Build history of the part. All positions in model axes, mm. A direction names the side the tool comes from. Round coordinates to 2 decimals unless told otherwise and drop trailing zeros. Order: outer loops, then holes, each group sorted by start corner. A loop starts at its lowest first (then second) coordinate and runs counter-clockwise, first axis right, second up. Notation, with made-up numbers: (-34.5, 43.25) -> (-11.5, 43.25) arc R30 cw to (-11.5, 75.25) -> close; hole circle Ø7 at (-23.75, 33). An arc over 180 degrees is marked (long way). Answer as a JSON object with one key per item and string values.
from build123d import *

# Parameters (mm, degrees)
F0_R     = 2.9
F1_DEPTH = 10
F2_W     = 29.9
F2_H     = 90
F3_DEPTH = 40
F4_W     = 7.6
F4_H     = 90
F5_DEPTH = 25
F6_R     = 3.4
F7_DEPTH = 30
F8_SIZE2 = 4
F8_SIZE  = 3


with BuildPart() as f1:
    # F0 (on Right) → F1 (new body)
    with BuildSketch(Plane.YZ):
        with BuildLine():
            Line((-75, -45), (75, -45))
            ThreePointArc((75, -45), (78.535534, -43.535534), (80, -40))
            Line((80, -40), (80, -10))
            ThreePointArc((80, -10), (78.535534, -6.464466), (75, -5))
            Line((75, -5), (45, -5))
            ThreePointArc((45, -5), (41.464466, -3.535534), (40, 0))
            Line((40, 0), (40, 40))
            ThreePointArc((40, 40), (38.535534, 43.535534), (35, 45))
            Line((35, 45), (-35, 45))
            ThreePointArc((-35, 45), (-38.535534, 43.535534), (-40, 40))
            Line((-40, 40), (-40, 0))
            ThreePointArc((-40, 0), (-41.464466, -3.535534), (-45, -5))
            Line((-45, -5), (-75, -5))
            ThreePointArc((-75, -5), (-78.535534, -6.464466), (-80, -10))
            Line((-80, -10), (-80, -40))
            ThreePointArc((-80, -40), (-78.535534, -43.535534), (-75, -45))
        make_face()
        with Locations((-65, -25)):
            Circle(F0_R, mode=Mode.SUBTRACT)
        with Locations((-25, -25)):
            Circle(F0_R, mode=Mode.SUBTRACT)
        with Locations((25, -25)):
            Circle(F0_R, mode=Mode.SUBTRACT)
        with Locations((65, -25)):
            Circle(F0_R, mode=Mode.SUBTRACT)
        with Locations((-25, 25)):
            Circle(F0_R, mode=Mode.SUBTRACT)
        with Locations((25, 25)):
            Circle(F0_R, mode=Mode.SUBTRACT)
    extrude(amount=F1_DEPTH)

    # F2 (on face) → F3 (join)
    with BuildSketch(Plane(origin=(0, 0, 0), x_dir=(0, -1, 0), z_dir=(-1, 0, 0))):
        Rectangle(F2_W, F2_H)
    extrude(amount=F3_DEPTH)

    # F4 (on face) → F5 (cut)
    with BuildSketch(Plane(origin=(-40, 0, 0), x_dir=(0, -1, 0), z_dir=(-1, 0, 0))):
        with Locations((-11.15, 0)):
            Rectangle(F4_W, F4_H)
        with Locations((11.15, 0)):
            Rectangle(F4_W, F4_H)
    extrude(amount=-F5_DEPTH, mode=Mode.SUBTRACT)

    # F6 (on face) → F7 (cut)
    with BuildSketch(Plane(origin=(-40, 0, 0), x_dir=(0, -1, 0), z_dir=(-1, 0, 0))):
        with Locations((0, 25)):
            Circle(F6_R)
        with Locations((0, -25)):
            Circle(F6_R)
    extrude(amount=-F7_DEPTH, mode=Mode.SUBTRACT)

    # F8
    f8_edges = [f1.edges().sort_by_distance(p)[0] for p in [
        (0, 22.1, 25),
        (0, -27.9, 25),
        (0, -67.9, -25),
        (0, -27.9, -25),
        (0, 22.1, -25),
        (0, 62.1, -25),
    ]]
    chamfer(f8_edges, length=F8_SIZE, length2=F8_SIZE2)


solid = f1.part
1) Cut at A-A, the plane y = -25. Give the cut face in (x, z), plus the area to 3 significant figures.
Checked values:
{"outline": "(0, -45) -> (10, -45) -> (10, -27.9) -> (4, -27.9) -> (0, -30.9) -> close; (0, -19.1) -> (4, -22.1) -> (10, -22.1) -> (10, 22.1) -> (4, 22.1) -> (0, 19.1) -> close; (0, 30.9) -> (4, 27.9) -> (10, 27.9) -> (10, 45) -> (0, 45) -> close", "area": "760 mm²"}
2) Cut at B-B, the plane z = 25. Give the cut face in (x, y), plus the area to 3 significant figures.
Checked values:
{"outline": "(-40, -7.35) -> (-15, -7.35) -> (-15, -14.95) -> (0, -14.95) -> (0, -19.1) -> (4, -22.1) -> (10, -22.1) -> (10, 22.1) -> (4, 22.1) -> (0, 19.1) -> (0, 14.95) -> (-15, 14.95) -> (-15, 7.35) -> (-40, 7.35) -> (-40, 3.4) -> (-10, 3.4) -> (-10, -3.4) -> (-40, -3.4) -> close; (0, -40) -> (10, -40) -> (10, -27.9) -> (4, -27.9) -> (0, -30.9) -> close; (0, 30.9) -> (4, 27.9) -> (10, 27.9) -> (10, 40) -> (0, 40) -> close", "area": "1,270 mm²"}
3) Flat gauge pins, fed straight in: pin 1 Ø4.5 at (x, z) = (-10, 18) entering from -Y; pin 2 Ø4.5 at (y, z) = (-25, 25) entering from -X; pin 3 Ø7.5 at (y, z) = (65, -25) entering from -X; pin 4 Ø8 at (x, y) = (6, 62.5) entering from +Z. Where does each tip first touch, or does it go through?
Checked values:
{"pin 1": "stops at y = -14.95", "pin 2": "passes through", "pin 3": "stops at x = 2.87", "pin 4": "stops at z = -5"}
4) Probe L1, parallel to Z at x = 6, y = -25; L2, parallel to Z at x = 5.2, y = -65; L3, parallel to X at y = -58.5, z = -22.5. List the from-to ranges inside material, lowest first. Write a range as from..to.
Checked values:
{"L1": "z = -45..-27.9, -22.1..22.1, 27.9..45", "L2": "z = -45..-27.9, -22.1..-5", "L3": "x = 0..10"}
5) Cut at D-D, the plane x = -35. Give the cut face in (y, z), plus the area to 3 significant figures.
Checked values:
{"outline": "(-7.35, -45) -> (7.35, -45) -> (7.35, 45) -> (-7.35, 45) -> close; hole circle Ø6.8 at (0, -25); hole circle Ø6.8 at (0, 25)", "area": "1,250 mm²"}
6) Cut at C-C, the plane y = -65. Give the cut face in (x, z), plus the area to 3 significant figures.
Checked values:
{"outline": "(0, -45) -> (10, -45) -> (10, -27.9) -> (4, -27.9) -> (0, -30.9) -> close; (0, -19.1) -> (4, -22.1) -> (10, -22.1) -> (10, -5) -> (0, -5) -> close", "area": "330 mm²"}
7) Pull direction Z, two halves, no side cores. Call faces 1 (the face through (5, 78, -44)), 2 (the face through (6.96, -62.32, -26.11)), 3 (the face through (5, -60, -5)), 4 (the face through (0, 40, -9)): pulls with the +Z half, pulls with the -Z half, needs draft (parallel to the pull), parting line crosses it, or undercut.
Checked values:
{"face 1": "pulls with the -Z half", "face 2": "undercut", "face 3": "pulls with the +Z half", "face 4": "needs draft"}
8) Which spindle directions (+Z, -Z, +X, -X, +Y, -Y) get a long thin tool onto all of the face, cutting with end or side? Do faces 5 (the face through (-25.21, 0.44, -21.63)), 6 (the face through (5, 60, -5)), 7 (the face through (-7, -14.95, -1)), 8 (the face through (5, -40, 20)), 9 (the face through (-15, 11, 1)). Say none if no direction does.
Checked values:
{"face 5": "-X", "face 6": "+Z, +X, -X, +Y", "face 7": "+Z, -Z, -X, -Y", "face 8": "+Z, +X, -X, -Y", "face 9": "+Z, -Z, -X, +Y"}
